from build123d import *

# Parameters (mm, degrees)
SKETCH1_W               = 19.05
SKETCH1_H               = 31.399999938
BOSS_EXTRUDE1_DEPTH     = 3
FILLET1_R               = 3.175
CUT_EXTRUDE1_DEPTH      = 28.507101338
CUT_EXTRUDE1_DEPTH_BACK = 28.507101338
SKETCH2_R               = 1.5


with BuildPart() as part:
    # Sketch1 → Boss-Extrude1 (new, symmetric)
    with BuildSketch(Plane.XY):
        Rectangle(SKETCH1_W, SKETCH1_H)
        Polygon((9.525, 15.699999969), (9.525, 9.699999969), (21.775, 9.699999969), (21.775, 15.699999969), (18.6, 15.699999969), (18.6, 12.699999969), (15.425, 12.699999969), (15.425, 15.699999969), align=None)
        Polygon((9.525, -15.699999969), (15.425, -15.699999969), (15.425, -12.699999969), (18.6, -12.699999969), (18.6, -15.699999969), (21.775, -15.699999969), (21.775, -9.699999969), (9.525, -9.699999969), align=None)
    extrude(amount=BOSS_EXTRUDE1_DEPTH, both=True)

    # Fillet1
    fillet1_edges = [part.edges().sort_by_distance(p)[0] for p in [
        (-9.525, -15.699999969, 0),
        (-9.525, 15.699999969, 0),
    ]]
    fillet(fillet1_edges, radius=FILLET1_R)

    # Sketch2 → Cut-Extrude1 (cut, two sides: drawn at the far end of the back side and taken through both)
    with BuildSketch(Plane.XY.offset(3).offset(-CUT_EXTRUDE1_DEPTH_BACK)):
        with Locations((0, 9.525)):
            Circle(SKETCH2_R)
        with Locations((0, -9.525)):
            Circle(SKETCH2_R)
        Circle(SKETCH2_R)
    extrude(amount=CUT_EXTRUDE1_DEPTH + CUT_EXTRUDE1_DEPTH_BACK, mode=Mode.SUBTRACT)


solid = part.part
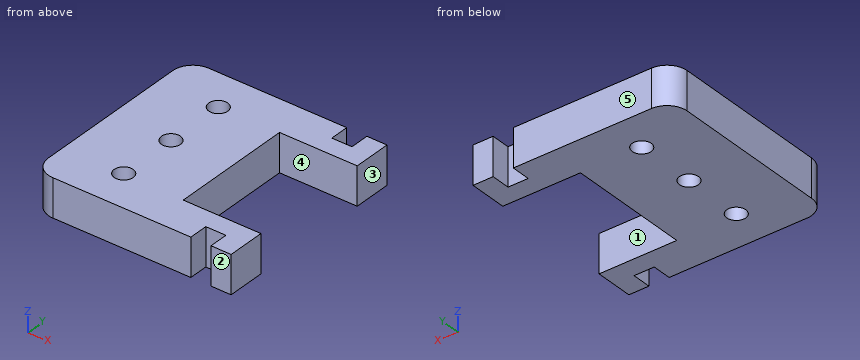
Could you check a few things on this model? Use its own coordinates, in mm. Face numbers are marked on the shaded views. A direction names the side the tool comes from. Round coordinates to 2 decimals unless told otherwise and drop trailing zeros. Order: outer loops, then holes, each group sorted by start corner. A loop starts at its lowest first (then second) coordinate and runs counter-clockwise, first axis right, second up. Notation, with made-up numbers: M 42.25,18 L 49.25,18 A28 cw 49.25,55 Z; hole C 52.5,-3 d6. An arc over 180 degrees is marked long. One line per item, written item: value.
(1) Imagine slicing it at C-C (z = -1.3). Write out the boundary of the cut face in (x, y) (3 decimals), and give its area (3 significant figures).
Ans:
outline: M -9.525,-12.525 A3.175 ccw -6.35,-15.7 L 15.425,-15.7 L 15.425,-12.7 L 18.6,-12.7 L 18.6,-15.7 L 21.775,-15.7 L 21.775,-9.7 L 9.525,-9.7 L 9.525,9.7 L 21.775,9.7 L 21.775,15.7 L 18.6,15.7 L 18.6,12.7 L 15.425,12.7 L 15.425,15.7 L -6.35,15.7 A3.175 ccw -9.525,12.525 Z; hole C 0,-9.525 d3; hole C 0,0 d3; hole C 0,9.525 d3
area: 701 mm^2
(2) I need wall thicknesses on line 1 along Y through (x, z) = (0, 0.1) (3 decimals); line 2 along X through (y, z) = (0, -1.8) (3 decimals); line 3 along Y through (x, z) = (18, 1.25). Which ranges of each line are inside material? Lowest first, please. Write a range as from..to.
Ans:
line 1: y = -15.7..-11.025, -8.025..-1.5, 1.5..8.025, 11.025..15.7
line 2: x = -9.525..-1.5, 1.5..9.525
line 3: y = -12.7..-9.7, 9.7..12.7
(3) Imagine slicing it at A-A (x = 14.5). Write out the boundary of the cut face in (y, z).
Ans:
outline: M -15.7,-3 L -9.7,-3 L -9.7,3 L -15.7,3 Z; M 9.7,-3 L 15.7,-3 L 15.7,3 L 9.7,3 Z
(4) Imagine slicing it at B-B (y = 0). Write out the boundary of the cut face in (x, z) (3 decimals), and give its area (3 significant figures).
Ans:
outline: M -9.525,-3 L -1.5,-3 L -1.5,3 L -9.525,3 Z; M 1.5,-3 L 9.525,-3 L 9.525,3 L 1.5,3 Z
area: 96.3 mm^2
(5) I'm going to push flat-ended pins straight in: P1, Ø5, axis at x = 0, y = 0, coming from the -Z side; P2, Ø1.5, axis at y = -14, z = 1, coming from the -X side; P3, Ø2.5, axis at y = 15, z = -1, coming from the -X side; P4, Ø1.6, axis at x = 17.5, z = 0.5, coming from the +Y side. Where does each tip first touch, or does it pass through?
Ans:
P1: stops at z = -3
P2: stops at x = -9.44
P3: stops at x = -9.28
P4: stops at y = 12.7
(6) If we mould it in two halves opening along Y, with no side actions, what happens to the marked faces 1, 2 and 3? For each: released by +Y, released by -Y, zero draft, split by the parting line, or undercut.
Ans:
face 1: undercut
face 2: released by -Y
face 3: zero draft
(7) Which directions (+Z, -Z, +X, -X, +Y, -Y) give clear straight access to the entire face, cutting with the end or side of a thin tool? Please do the marked faces 4 and 5.
Ans:
face 4: +Z, -Z, +X
face 5: +Z, -Z, +X, -X, +Y
(8) Imagine slicing it at D-D (x = 0). Write out the boundary of the cut face in (y, z) (3 decimals).
Ans:
outline: M -15.7,-3 L -11.025,-3 L -11.025,3 L -15.7,3 Z; M -8.025,-3 L -1.5,-3 L -1.5,3 L -8.025,3 Z; M 1.5,-3 L 8.025,-3 L 8.025,3 L 1.5,3 Z; M 11.025,-3 L 15.7,-3 L 15.7,3 L 11.025,3 Z
